Here's how the part is built. I have some questions about the finished solid (model axes, mm). Face numbers are marked on the shaded views. A direction names the side the tool comes from. Coordinates: 2 decimals unless noted, no trailing zeros. Loops run counter-clockwise (first coordinate to the right, second up) from the corner with the lowest first, then second, coordinate; pieces in that order, holes last. Notation, with made-up numbers: (45, 43.25) -> (65, 43.25) arc R12 cw to (65, 47.25) -> close; hole circle Ø3 at (23.25, 39). An arc over 180 degrees is marked (long way). Answer as a JSON object with one key per item and string values. Group by question number.
Q1. I need wall thicknesses on line 1 (Z direction, x = 2.45, y = 5); line 2 (Z direction, x = 3, y = 6.75); line 3 (Z direction, x = 6.5, y = 5). Which ranges of each line are inside material? Lowest first, please.
Q2. I want a section at D-D on z = -33.75. Write out the boundary of the cut face in (x, y).
Q3. I want a section at C-C on y = 5. Write out the boundary of the cut face in (x, z), then the cut area to 3 significant figures.
Q4. I want a section at B-B on x = 4.25. Write out the boundary of the cut face in (y, z), then the cut area to 3 significant figures.
Q5. On a 3-axis mill with a long thin cutter (end or side, diameter ignored), from which of +Z, -Z, +X, -X, +Y, -Y can I reach the whole of each face in a straight line? I mean the marked faces 1, 2, 3 and 4. Say none if no direction works.
Q6. I'm going to push flat-ended pins straight in: pin 1 (4 mm diameter, centred on x = 2, z = -9, fed in from -Y); pin 2 (4 mm diameter, centred on y = 5, z = -33.75, fed in from -X); pin 3 (1.5 mm diameter, centred on x = 1.5, z = -15.5, fed in from +Y); pin 4 (2.5 mm diameter, centred on x = 7.5, y = 4.5, fed in from +Z). Where does each tip first touch, or does it pass through?
Q7. I want a section at A-A on z = -19.5. Write out the boundary of the cut face in (x, y), then the cut area to 3 significant figures.
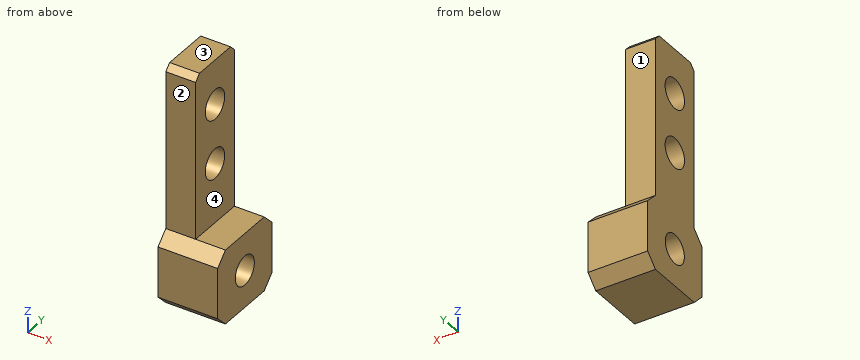
Autodesk Inventor part; units mm, degrees
ref_plane "YZ Plane" through (0, 0, 0) normal (1, 0, 0) x (0, 1, 0)
ref_plane "XZ Plane" through (0, 0, 0) normal (0, 1, 0) x (-1, 0, 0)
ref_plane "XY Plane" through (0, 0, 0) normal (0, 0, 1) x (1, 0, 0)
sketch "Sketch1" plane through (0, 0, 0) normal (1, 0, 0) x (0, 1, 0)
  circle A0 centre (5, -7.5) radius 2.5
  circle A1 centre (5, -17.5) radius 2.5
  line L0 (0, -30) -> (10, -30)
  line L1 (10, -30) -> (10, 0)
  line L2 (10, 0) -> (0, 0)
  line L3 (0, 0) -> (0, -30)
  dimension "d23" = 30
  dimension "d25" = 30
  dimension "d38" = 10
  dimension "d39" = 5
  dimension "d40" = 5
  dimension "d41" = 10
  dimension "d42" = 5
  dimension "d43" = 5
extrude "Extrusion1" add sketch "Sketch1" along normal blind 5
sketch "Sketch2" plane through (0, 0, -30) normal (0, 0, -1) x (-1, 0, 0)
  line L0 (0, 0) -> (0, 10)
  line L1 (0, 10) -> (-5, 10)
  line L2 (-5, 0) -> (-5, 10)
  line L3 (0, 0) -> (-5, 0)
extrude "Extrusion2" add sketch "Sketch2" along normal blind 10
sketch "Sketch4" plane through (0, 10, 0) normal (0, 1, 0) x (1, 0, 0)
  line L0 (5, 0) -> (5, 40)
  line L1 (0, 40) -> (5, 40)
  line L2 (0, 40) -> (5, 40)
  line L3 (5, 40) -> (5, 27.5)
  line L4 (5, 27.5) -> (0, 27.5)
  line L5 (0, 27.5) -> (0, 40)
  dimension "d5" = 12.5
extrude "Extrusion3" add sketch "Sketch4" along normal blind 2
sketch "Sketch5" plane through (0, 0, 0) normal (0, -1, 0) x (1, 0, 0)
  line L0 (5, 0) -> (5, -40)
  line L1 (0, -40) -> (5, -40)
  line L2 (5, -40) -> (5, -27.5)
  line L3 (5, -27.5) -> (0, -27.5)
  line L4 (0, -27.5) -> (0, -40)
  dimension "d8" = 12.5
extrude "Extrusion4" add sketch "Sketch5" along normal blind 2
sketch "Sketch6" plane through (5, 0, 0) normal (1, 0, 0) x (0, 0, -1)
  line L0 (27.5, 12) -> (40, 12)
  line L1 (40, 12) -> (40, -2)
  line L2 (40, -2) -> (27.5, -2)
  line L3 (27.5, -2) -> (27.5, 12)
  line L4 (40, -2) -> (40, 12)
  line L5 (27.5, 12) -> (40, 12)
chamfer "Chamfer3" distance 1 angle 45 2 edges at (2.5, 10, 0) (2.5, 0, 0)
extrude "Extrusion6" add sketch "Sketch6" along normal blind 5
chamfer "Chamfer4" distance 2 angle 45 4 edges at (5, 12, -27.5) (5, 12, -40) (5, -2, -40) (5, -2, -27.5)
sketch "Sketch7" plane through (10, 0, 0) normal (1, 0, 0) x (0, 0, -1)
  line L0 (40, 0) -> (40, 10)
  line L1 (38, 12) -> (29.5, 12)
  point P0 (0, 0)
  point P1 (33.75, 5)
  dimension "d44" = 7
  dimension "d45" = 6.25
hole "Hole1" at (10, 5, -33.75) direction (-1, 0, 0) diameter 4.917 end through all
properties part number "holder"
Result set:
{
 "1": {"line 1": "z = -40 to -36.21, -31.29 to -20, -15 to -10, -5 to 0", "line 2": "z = -40 to -35.48, -32.02 to -19.29, -15.71 to -9.29, -5.71 to 0", "line 3": "z = -40 to -36.21, -31.29 to -27.5"},
 "2": {"outline": "(0, -2) -> (10, -2) -> (10, 2.54) -> (0, 2.54) -> close; (0, 7.46) -> (10, 7.46) -> (10, 12) -> (0, 12) -> close"},
 "3": {"outline": "(0, -40) -> (10, -40) -> (10, -36.21) -> (0, -36.21) -> close; (0, -31.29) -> (10, -31.29) -> (10, -27.5) -> (5, -27.5) -> (5, -20) -> (0, -20) -> close; (0, -15) -> (5, -15) -> (5, -10) -> (0, -10) -> close; (0, -5) -> (5, -5) -> (5, 0) -> (0, 0) -> close", "area": "163 mm²"},
 "4": {"outline": "(-2, -38) -> (0, -40) -> (10, -40) -> (12, -38) -> (12, -29.5) -> (10, -27.5) -> (10, -1) -> (9, 0) -> (1, 0) -> (0, -1) -> (0, -27.5) -> (-2, -29.5) -> close; hole circle Ø5 at (5, -17.5); hole circle Ø5 at (5, -7.5); hole circle Ø4.92 at (5, -33.75)", "area": "383 mm²"},
 "5": {"face 1": "+Z, +X, -X, +Y", "face 2": "+Z, +X, -X, -Y", "face 3": "+Z, +X, -X, +Y, -Y", "face 4": "+Z, +X, +Y, -Y"},
 "6": {"pin 1": "stops at y = 0", "pin 2": "passes through", "pin 3": "stops at y = 10", "pin 4": "stops at z = -27.5"},
 "7": {"outline": "(0, 0) -> (5, 0) -> (5, 3.5) -> (0, 3.5) -> close; (0, 6.5) -> (5, 6.5) -> (5, 10) -> (0, 10) -> close", "area": "35.0 mm²"}
}
